Read the model definition and answer for the solid it produces. Units are mm, in the model's axes. Give positions to 0.01 mm unless a question says otherwise; leave off trailing zeros. Order: outer loops, then holes, each group sorted by start corner. A loop starts at its lowest first (then second) coordinate and runs counter-clockwise, first axis right, second up. Notation, with made-up numbers: (39, 19.25) - (45, 19.25) arc R10 ccw to (45, 24.25) - close; hole circle Ø7 at (63, 47.25). An arc over 180 degrees is marked (long way). Write item = value, one per line.
```python
from build123d import *

# Parameters (mm, degrees)
BOSS_EXTRUDE1_DEPTH      = 5.07492
SKETCH6_R                = 22.225
BOSS_EXTRUDE3_DEPTH      = 5.07492
SKETCH2_3_R              = 6.35
CUT_EXTRUDE2_DEPTH       = 5.588
SKETCH8_W                = 2.728150378
SKETCH8_H                = 127
BOSS_EXTRUDE4_DEPTH      = 5.07492
SKETCH9_W                = 3.563296166
SKETCH9_H                = 127
BOSS_EXTRUDE5_DEPTH      = 5.07492
SKETCH12_R               = 3
CUT_EXTRUDE3_DEPTH       = 400.05
SKETCH13_3_R             = 2
CUT_EXTRUDE10_DEPTH      = 1549.4
SKETCH15_R               = 2.9972
CUT_EXTRUDE11_DEPTH      = 1549.4
SKETCH13_4_R             = 6.35
CUT_EXTRUDE12_DEPTH      = 1549.4
CUT_EXTRUDE13_START      = 223.266
SKETCH13_R               = 22.86
SKETCH13_R_2             = 2
SKETCH13_R_3             = 6.35
CUT_EXTRUDE13_DEPTH      = 1549.4
CUT_EXTRUDE14_DEPTH      = 2.54
CUT_EXTRUDE14_DEPTH_BACK = 6.35
SKETCH16_R               = 1.524
SKETCH17_R               = 1.905
CUT_EXTRUDE15_DEPTH      = 6.35
SKETCH18_R               = 2.159
SKETCH18_R_2             = 3.175
SKETCH18_R_3             = 2.286
CUT_EXTRUDE16_DEPTH      = 6.35


with BuildPart() as part:
    # Sketch2 → Boss-Extrude1 (new body)
    with BuildSketch(Plane.XY):
        with BuildLine():
            Line((-143.383, -31.75), (-127.127, -31.75))
            ThreePointArc((-127.127, -31.75), (-123.317, -30.48), (-119.507, -31.75))
            Line((-119.507, -31.75), (119.253, -31.75))
            ThreePointArc((119.253, -31.75), (123.063, -30.48), (126.873, -31.75))
            Line((126.873, -31.75), (143.383, -31.75))
            Line((143.383, -31.75), (143.383, 95.25))
            Line((143.383, 95.25), (-143.383, 95.25))
            Line((-143.383, 95.25), (-143.383, -31.75))
        make_face()
    extrude(amount=-BOSS_EXTRUDE1_DEPTH)

    # Sketch6 → Boss-Extrude3 (add)
    with BuildSketch(Plane(origin=(0, 0, -5.07492), x_dir=(-1, 0, 0), z_dir=(0, 0, -1))):
        with Locations((-123.063, -36.83)):
            Circle(SKETCH6_R)
        with Locations((123.317, -36.83)):
            Circle(SKETCH6_R)
    extrude(amount=-BOSS_EXTRUDE3_DEPTH)

    # Sketch2_3 → Cut-Extrude2 (cut)
    with BuildSketch(Plane.XY):
        with Locations((-123.317, -36.83)):
            Circle(SKETCH2_3_R)
        with Locations((123.063, -36.83)):
            Circle(SKETCH2_3_R)
    extrude(amount=-CUT_EXTRUDE2_DEPTH, mode=Mode.SUBTRACT)

    # Sketch8 → Boss-Extrude4 (add)
    with BuildSketch(Plane(origin=(0, 0, -5.07492), x_dir=(-1, 0, 0), z_dir=(0, 0, -1))):
        with Locations((144.139824811, 31.75)):
            Rectangle(SKETCH8_W, SKETCH8_H)
    extrude(amount=-BOSS_EXTRUDE4_DEPTH)

    # Sketch9 → Boss-Extrude5 (add)
    with BuildSketch(Plane(origin=(0, 0, -5.07492), x_dir=(-1, 0, 0), z_dir=(0, 0, -1))):
        with Locations((-145.164648083, 31.75)):
            Rectangle(SKETCH9_W, SKETCH9_H)
    extrude(amount=-BOSS_EXTRUDE5_DEPTH)

    # Sketch12 → Cut-Extrude3 (cut)
    with BuildSketch(Plane.XY):
        with Locations((-123.317, 76.2)):
            Circle(SKETCH12_R)
        with Locations((123.063, 76.2)):
            Circle(SKETCH12_R)
    extrude(amount=-CUT_EXTRUDE3_DEPTH, mode=Mode.SUBTRACT)


with BuildPart() as body_2:
    # Mirror1: mirrored copy
    add(part.part.mirror(Plane(origin=(0, 0, -114.29492), x_dir=(1, 0, 0), z_dir=(0, 0, -1))))

    # Sketch13_3 → Cut-Extrude10 (cut)
    with BuildSketch(Plane(origin=(0, 0, -5.07492), x_dir=(-1, 0, 0), z_dir=(0, 0, -1))):
        with Locations((23.390611843, 18.7706)):
            Circle(SKETCH13_3_R)
        with Locations((5.890011843, 1.27)):
            Circle(SKETCH13_3_R)
        with Locations((40.891211843, 1.27)):
            Circle(SKETCH13_3_R)
        with Locations((23.390611843, -16.2306)):
            Circle(SKETCH13_3_R)
        with Locations((-32.258, 67.0306)):
            Circle(SKETCH13_3_R)
        with Locations((-14.7574, 49.53)):
            Circle(SKETCH13_3_R)
        with Locations((-32.258, 32.0294)):
            Circle(SKETCH13_3_R)
        with Locations((-49.7586, 49.53)):
            Circle(SKETCH13_3_R)
    extrude(amount=CUT_EXTRUDE10_DEPTH, mode=Mode.SUBTRACT)

    # Sketch15 → Cut-Extrude11 (cut)
    with BuildSketch(Plane.XY.offset(-223.51492)):
        with Locations((-87.0839, -19.05)):
            Circle(SKETCH15_R)
        with Locations((86.868, -19.05)):
            Circle(SKETCH15_R)
    extrude(amount=-CUT_EXTRUDE11_DEPTH, mode=Mode.SUBTRACT)

    # Sketch13_4 → Cut-Extrude12 (cut)
    with BuildSketch(Plane(origin=(0, 0, -5.07492), x_dir=(-1, 0, 0), z_dir=(0, 0, -1))):
        with Locations((23.390611843, 1.27)):
            Circle(SKETCH13_4_R)
        with Locations((-32.258, 49.53)):
            Circle(SKETCH13_4_R)
    extrude(amount=CUT_EXTRUDE12_DEPTH, mode=Mode.SUBTRACT)

    # Sketch13 → Cut-Extrude13 (cut)
    # profile 1 of 2: a face of its own
    with BuildSketch(Plane(origin=(0, 0, -5.07492), x_dir=(-1, 0, 0), z_dir=(0, 0, -1)).offset(CUT_EXTRUDE13_START)):
        with Locations((23.390611843, 1.27)):
            Circle(SKETCH13_R)
        with Locations((23.390611843, 18.7706)):
            Circle(SKETCH13_R_2, mode=Mode.SUBTRACT)
        with Locations((40.891211843, 1.27)):
            Circle(SKETCH13_R_2, mode=Mode.SUBTRACT)
        with Locations((23.390611843, -16.2306)):
            Circle(SKETCH13_R_2, mode=Mode.SUBTRACT)
        with Locations((5.890011843, 1.27)):
            Circle(SKETCH13_R_2, mode=Mode.SUBTRACT)
        with Locations((23.390611843, 1.27)):
            Circle(SKETCH13_R_3, mode=Mode.SUBTRACT)
    # profile 2 of 2: a face of its own
    with BuildSketch(Plane(origin=(0, 0, -5.07492), x_dir=(-1, 0, 0), z_dir=(0, 0, -1)).offset(CUT_EXTRUDE13_START)):
        with Locations((-32.258, 49.53)):
            Circle(SKETCH13_R)
        with Locations((-32.258, 67.0306)):
            Circle(SKETCH13_R_2, mode=Mode.SUBTRACT)
        with Locations((-14.7574, 49.53)):
            Circle(SKETCH13_R_2, mode=Mode.SUBTRACT)
        with Locations((-32.258, 32.0294)):
            Circle(SKETCH13_R_2, mode=Mode.SUBTRACT)
        with Locations((-49.7586, 49.53)):
            Circle(SKETCH13_R_2, mode=Mode.SUBTRACT)
        with Locations((-32.258, 49.53)):
            Circle(SKETCH13_R_3, mode=Mode.SUBTRACT)
    extrude(amount=CUT_EXTRUDE13_DEPTH, mode=Mode.SUBTRACT)

    # Sketch16 → Cut-Extrude14 (cut, two sides: drawn at the far end of the back side and taken through both)
    with BuildSketch(Plane.XY.offset(-223.51492).offset(-CUT_EXTRUDE14_DEPTH_BACK)):
        with Locations(Location((2.007444266, 44.229302642, 0), (0, 0, 180))):
            Circle(SKETCH16_R)
        with Locations(Location((11.683653899, 26.728907983, 0), (0, 0, 180))):
            Circle(SKETCH16_R)
        with Locations(Location((52.832346101, 26.728907983, 0), (0, 0, 180))):
            Circle(SKETCH16_R)
        with Locations(Location((62.486930452, 44.107336595, 0), (0, 0, 180))):
            Circle(SKETCH16_R)
        with Locations(Location((-53.618108667, -4.286724908, 0), (0, 0, 180))):
            Circle(SKETCH16_R)
        with Locations(Location((-43.83565651, -21.677307131, 0), (0, 0, 180))):
            Circle(SKETCH16_R)
        with Locations(Location((-2.945567175, -21.677307131, 0), (0, 0, 180))):
            Circle(SKETCH16_R)
        with Locations(Location((6.836884982, -4.286724908, 0), (0, 0, 180))):
            Circle(SKETCH16_R)
    extrude(amount=CUT_EXTRUDE14_DEPTH + CUT_EXTRUDE14_DEPTH_BACK, mode=Mode.SUBTRACT)

    # Sketch17 → Cut-Extrude15 (cut)
    with BuildSketch(Plane.XY.offset(-223.51492)):
        with Locations((-131.474681475, -8.33115872)):
            Circle(SKETCH17_R)
        with Locations((-115.059944142, -8.33115872)):
            Circle(SKETCH17_R)
        with Locations((-123.317, -35.561808249)):
            Circle(SKETCH17_R)
        with Locations((123.063, -35.433)):
            Circle(SKETCH17_R)
        with Locations((114.346312611, -8.247692484)):
            Circle(SKETCH17_R)
        with Locations((131.954972652, -8.247692484)):
            Circle(SKETCH17_R)
    extrude(amount=-CUT_EXTRUDE15_DEPTH, mode=Mode.SUBTRACT)

    # Sketch18 → Cut-Extrude16 (cut)
    with BuildSketch(Plane.XY.offset(-223.51492)):
        with Locations((-48.522954976, -21.971)):
            Circle(SKETCH18_R)
        with Locations((4.033472896, -22.225)):
            Circle(SKETCH18_R_2)
        with Locations((67.080879188, 15.068285327)):
            Circle(SKETCH18_R_3)
    extrude(amount=-CUT_EXTRUDE16_DEPTH, mode=Mode.SUBTRACT)


solid = body_2.part
```
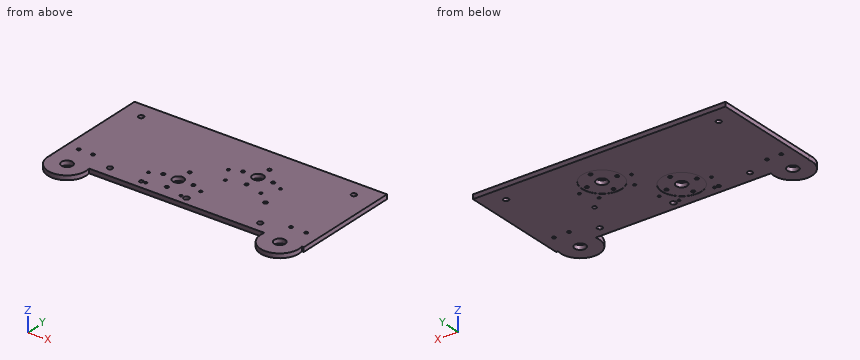
1. Section B-B (y = 76.2) is taken. Determine the outline of the cut face in (x, z), and give its area (3 significant figures).
Recorded:
outline = (-145.5, -228.59) - (-126.32, -228.59) - (-126.32, -223.51) - (-145.5, -223.51) - close; (-120.32, -228.59) - (120.06, -228.59) - (120.06, -223.51) - (-120.32, -223.51) - close; (126.06, -228.59) - (146.95, -228.59) - (146.95, -223.51) - (126.06, -223.51) - close
area = 1,420 mm^2
2. Section D-D (z = -227.05) is taken. Count the separate pieces of the cut face and the enclosed holes in it, and give its area (3 significant figures).
Recorded:
separate_pieces = 1
enclosed_holes = 31
area = 38,300 mm^2
3. Flat-ended cylindrical pins translate along their axes: pin 1 (6.5 mm diameter, centred on x = -5.89, y = 1.27, fed in from -Z); pin 2 (2 mm diameter, centred on y = 2, z = -227, fed in from -X); pin 3 (2 mm diameter, centred on x = -9.5, z = -226, fed in from -Y). Find the tip coordinate at first contact, or state that the pin passes through.
Recorded:
pin_1 = -228.34
pin_2 = -145.5
pin_3 = -31.75
4. Section A-A (y = -36.83) is taken. Determine the outline of the cut face in (x, z).
Recorded:
outline = (-145.54, -228.59) - (-129.67, -228.59) - (-129.67, -223.51) - (-145.54, -223.51) - close; (-116.97, -228.59) - (-101.09, -228.59) - (-101.09, -223.51) - (-116.97, -223.51) - close; (100.84, -228.59) - (116.71, -228.59) - (116.71, -223.51) - (100.84, -223.51) - close; (129.41, -228.59) - (145.29, -228.59) - (145.29, -223.51) - (129.41, -223.51) - close
5. Straight lines are drawn through the part: L1, parallel to X at y = 49.53, z = -226.7; L2, parallel to X at y = 27, z = -227.5; L3, parallel to X at y = -41.5, z = -227.2. For each, find the intervals that lie inside material, in ascending order. Write a range as [from, to].
Recorded:
L1 = [-145.5, 12.76], [16.76, 25.91], [38.61, 47.76], [51.76, 146.95]
L2 = [-145.5, 10.18], [13.18, 51.33], [54.33, 146.95]
L3 = [-145.05, -127.62], [-119.01, -101.59], [101.33, 118.76], [127.37, 144.79]
6. Section C-C (x = -59) is taken. Determine the outline of the cut face in (y, z), and give its area (3 significant figures).
Recorded:
outline = (-31.75, -228.59) - (95.25, -228.59) - (95.25, -223.51) - (-31.75, -223.51) - close
area = 645 mm^2
